Design review of the part built by this model. Coordinates are the model's own, in mm. A direction names the side the tool comes from. Give positions to 0.01 mm unless a question says otherwise; leave off trailing zeros. Order: outer loops, then holes, each group sorted by start corner. A loop starts at its lowest first (then second) coordinate and runs counter-clockwise, first axis right, second up.
```python
from build123d import *

# Parameters (mm, degrees)
EXTRUDE_1_DEPTH     = 86
CUT_EXTRUDE_1_DEPTH = 3
EXTRUDE_2_DEPTH     = 10


with BuildPart() as part:
    # Эскиз1 → Бобышка-Вытянуть1 (new body)
    with BuildSketch(Plane.XY):
        Polygon((35, -4), (33, -4), (-35, 36), (-35, 38), align=None)
    extrude(amount=EXTRUDE_1_DEPTH)

    # Эскиз2 → Вырез-Вытянуть1 (cut)
    with BuildSketch(Plane(origin=(7.5, 12.5, 0), x_dir=(0.8574929257125444, -0.5144957554275262, 0), z_dir=(0.5144957554275262, 0.8574929257125444, 0))):
        Polygon((22.070235422, -3), (32.070235422, -3), (32.070235422, 0), (-49.563091106, 0), align=None)
        Polygon((-49.563091106, -21), (-49.563091106, -43), (22.038839221, -43), (2.070235422, -21), align=None)
        Polygon((-49.563091106, -43), (-49.563091106, -65), (2.070235422, -65), (22.038839221, -43), align=None)
        Polygon((22.070235422, -83), (-49.563091106, -86), (32.070235422, -86), (32.070235422, -83), align=None)
    extrude(amount=-CUT_EXTRUDE_1_DEPTH, mode=Mode.SUBTRACT)

    # Эскиз3 → Бобышка-Вытянуть2 (add)
    with BuildSketch(Plane(origin=(7.5, 12.5, 0), x_dir=(0.8574929257125444, -0.5144957554275262, 0), z_dir=(0.5144957554275262, 0.8574929257125444, 0))):
        Polygon((-49.563091106, -65), (-49.563091106, -86), (22.070235422, -83), (32.070235422, -83), (32.070235422, -81.5), (22.038839221, -81.5), (-48.063091106, -84.435865207), (-48.063091106, -66.5), (2.734491563, -66.5), (24.064591076, -43), (2.734491563, -19.5), (-48.063091106, -19.5), (-48.063091106, -1.564134793), (22.038839221, -4.5), (32.070235422, -4.5), (32.070235422, -3), (22.070235422, -3), (-49.563091106, 0), (-49.563091106, -21), (2.070235422, -21), (22.038839221, -43), (2.070235422, -65), align=None)
    extrude(amount=EXTRUDE_2_DEPTH)


solid = part.part
```
1. For pin 1 (4 mm diameter, centred on x = 5.5, y = 10.5, fed in from -Z); pin 2 (12 mm diameter, centred on y = 16.5, z = 64.5, fed in from +X); pin 3 (4 mm diameter, centred on x = -2.5, y = 29.5, fed in from +Z), all flat-tipped, find the tip position at first contact; note any pin that passes through.
Recorded:
pin 1: stops at z = 1.99
pin 2: stops at x = 21.2
pin 3: stops at z = 84.73
2. Take a section at A-A (z = 80). State the section outline as (x, y) points, then the cut area to 3 significant figures.
Recorded:
outline: (-35, 36) - (33, -4) - (35, -4) - (-33.71, 37.23) - (-28.57, 45.8) - (-29.86, 46.57) - (-35, 38) - close
area: 125 mm2
3. Take a section at C-C (y = 22.5). State the section outline as (x, z) points, then the cut area to 3 significant figures.
Recorded:
outline: (-12.05, 1.16) - (10.27, 1.96) - (10.27, 3.46) - (-9.17, 2.76) - (-9.17, 19.5) - (10.27, 19.5) - (10.27, 21) - (-12.05, 21) - close; (-12.05, 65) - (10.27, 65) - (10.27, 66.5) - (-9.17, 66.5) - (-9.17, 83.24) - (10.27, 82.54) - (10.27, 84.04) - (-12.05, 84.84) - close
area: 231 mm2
4. Take a section at B-B (x = 18). State the section outline as (y, z) points, then the cut area to 3 significant figures.
Recorded:
outline: (4.82, 2.62) - (17.86, 2.34) - (17.86, 3.84) - (6.2, 4.09) - (6.2, 29.98) - (17.86, 23.37) - (17.86, 25.6) - (4.82, 32.99) - close; (4.82, 53.01) - (17.86, 60.4) - (17.86, 62.63) - (6.2, 56.02) - (6.2, 81.91) - (17.86, 82.16) - (17.86, 83.66) - (4.82, 83.38) - close
area: 170 mm2
5. Machinability: for faces 4 (the face through (21.4, 9.91, 54.91)), 5 (the face through (33, 3, 81.5)), 6 (the face through (-35, 37, 75)), which of the approach directions +Z, -Z, +X, -X, +Y, -Y give a long, thin tool a straight path to every point of the face, cutting with its end or side? Answer none if there is none.
Recorded:
face 4: +X
face 5: +X, +Y
face 6: +Z, -Z, -X, +Y, -Y
6. For line 1 along Z through (x, y) = (-23, 40.5); line 2 along Z through (x, y) = (12.5, 10); line 3 along X through (y, z) = (7, 46), list the stretches that pass through material, from the lowest coordinate up.
Recorded:
line 1: z = 0.38 to 1.88, 19.5 to 21, 65 to 66.5, 84.12 to 85.62
line 2: z = 2.31 to 3.81, 22.63 to 24.86, 61.14 to 63.37, 82.19 to 83.69
line 3: x = 26.73 to 29.09
7. Draft analysis for pull direction Z (two halves, no side actions). For faces 1 (the face through (33, 2, 83)), 2 (the face through (-32.46, 42.23, 75.35)), 3 (the face through (-10, 29, 66.5)), state which applies: pulls with the +Z half, pulls with the -Z half, needs draft (parallel to the pull), parting line crosses it, or undercut.
Recorded:
face 1: pulls with the +Z half
face 2: needs draft
face 3: undercut
8. Take a section at D-D (y = 3). State the section outline as (x, z) points.
Recorded:
outline: (21.1, 2.77) - (27.54, 3) - (39.2, 3) - (39.2, 4.5) - (27.5, 4.5) - (23.33, 4.35) - (23.33, 36.83) - (29.86, 43) - (23.33, 49.17) - (23.33, 81.65) - (27.5, 81.5) - (39.2, 81.5) - (39.2, 83) - (27.54, 83) - (21.1, 83.23) - (21.1, 49.05) - (27.5, 43) - (21.1, 36.95) - close
